from build123d import *

# Parameters (mm, degrees)
F0_W     = 300
F0_H     = 24.5
F0_R     = 2.65
F1_DEPTH = 2
F2_DEPTH = 10
F3_DEPTH = 30
F4_R     = 1.7
F5_DEPTH = 2
F6_R     = 1.25
F7_DEPTH = 2


with BuildPart() as f1:
    # F0 (on Top) → F1 (new body)
    with BuildSketch(Plane.XY):
        Rectangle(F0_W, F0_H)
        with Locations((-75, 0)):
            Circle(F0_R, mode=Mode.SUBTRACT)
        with Locations((-60, 0)):
            Circle(F0_R, mode=Mode.SUBTRACT)
        with Locations((-45, 0)):
            Circle(F0_R, mode=Mode.SUBTRACT)
        with Locations((-30, 0)):
            Circle(F0_R, mode=Mode.SUBTRACT)
        with Locations((-15, 0)):
            Circle(F0_R, mode=Mode.SUBTRACT)
        Circle(F0_R, mode=Mode.SUBTRACT)
        with Locations((15, 0)):
            Circle(F0_R, mode=Mode.SUBTRACT)
        with Locations((30, 0)):
            Circle(F0_R, mode=Mode.SUBTRACT)
        with Locations((45, 0)):
            Circle(F0_R, mode=Mode.SUBTRACT)
        with Locations((60, 0)):
            Circle(F0_R, mode=Mode.SUBTRACT)
        with Locations((75, 0)):
            Circle(F0_R, mode=Mode.SUBTRACT)
    extrude(amount=F1_DEPTH)

    # F2 (add): a face of the model
    f2_faces = [f1.faces().sort_by_distance(p)[0] for p in [
        (-150, 0, 1),
    ]]
    extrude(f2_faces, amount=F2_DEPTH)

    # F3 (add): a face of the model
    f3_faces = [f1.faces().sort_by_distance(p)[0] for p in [
        (150, 0, 1),
    ]]
    extrude(f3_faces, amount=F3_DEPTH)

    # F4 (on face) → F5 (cut, through all)
    with BuildSketch(Plane.XY.offset(2)):
        with Locations((-153.6, 0)):
            Circle(F4_R)
    extrude(amount=-F5_DEPTH, mode=Mode.SUBTRACT)

    # F6 (on face) → F7 (cut, through all)
    with BuildSketch(Plane.XY.offset(2)):
        with Locations((158.75, -7.25)):
            Circle(F6_R)
    extrude(amount=-F7_DEPTH, mode=Mode.SUBTRACT)


solid = f1.part
Can you work these out from the model? Positions are in its coordinate system, mm. Give positions to 0.01 mm unless a question says otherwise; leave off trailing zeros. Write each question's results on one line, items separated by ' | '.
1) Suppose I cut it at A-A, the plane z = 0.4. Give the number of separate pieces and of enclosed holes in the cut face, then the cut area to 3 significant figures.
Final values:
separate pieces: 1 | enclosed holes: 13 | area: 8,070 mm^2
2) I'm going to push a flat-ended pin straight in: pin 1 Ø5 at (x, y) = (60, 0) entering from -Z. Where does the tip first touch, or does it pass through?
Final values:
pin 1: passes through
3) If we mould it in two halves opening along X, with no side actions, what happens to faces 1 (the face through (-72.472, 0.796, 0.986)), 2 (the face through (27.353, 0.117, 0.986)), 3 (the face through (8, 0, 2))? For each: pulls with the +X half, pulls with the -X half, needs draft (parallel to the pull), parting line crosses it, or undercut.
Final values:
face 1: undercut | face 2: undercut | face 3: needs draft
4) Please list where these lines run through material, in increasing order: line 1 along Y through (x, z) = (-153.6, 0.7); line 2 along Y through (x, z) = (-60, 0.7); line 3 along X through (y, z) = (-6.75, 1.5). Write a range as [from, to].
Final values:
line 1: y = [-12.25, -1.7], [1.7, 12.25] | line 2: y = [-12.25, -2.65], [2.65, 12.25] | line 3: x = [-160, 157.6], [159.9, 180]
